from build123d import *

# Parameters (mm, degrees)
BOSS_EXTRU_1_DEPTH                      = 7
ESQUISSE2_R                             = 4
ESQUISSE2_R_2                           = 1.2
BOSS_EXTRU_2_DEPTH                      = 7
CONG_1_R                                = 10
CONG_2_R                                = 3
DIAM_TRE_DU_PER_AGE_2_4_2_4_1_D         = 2.4
DIAM_TRE_DU_PER_AGE_2_4_2_4_1_ON_FACE_D = 2.4
DIAM_TRE_DU_PER_AGE_2_4_2_4_1_ON_F_2_D  = 2.4


with BuildPart() as part:
    # Esquisse1 → Boss.-Extru.1 (new body)
    with BuildSketch(Plane(origin=(0, 0, 0), x_dir=(1, 0, 0), z_dir=(0, 1, 0))):
        with BuildLine():
            Line((163.5, -54.314885969), (163.5, 54.839745962))
            Line((163.5, 54.839745962), (123.5, 124.121778265))
            Line((123.5, 124.121778265), (119.169872981, 121.621778265))
            Line((119.169872981, 121.621778265), (158.5, 53.5))
            Line((158.5, 53.5), (158.5, -53.5))
            ThreePointArc((158.5, -53.5), (146.077391865, -81.52236249), (128.750264504, -106.807627959))
            Line((128.750264504, -106.807627959), (132.598479772, -110))
            ThreePointArc((132.598479772, -110), (150.644566487, -83.59767596), (163.5, -54.314885969))
        make_face()
    extrude(amount=BOSS_EXTRU_1_DEPTH)

    # Esquisse2 → Boss.-Extru.2 (add)
    # profile 1 of 2: a face of its own
    with BuildSketch(Plane(origin=(0, 7, 0), x_dir=(1, 0, 0), z_dir=(0, 1, 0))):
        with Locations((155, 53)):
            Circle(ESQUISSE2_R)
        with Locations(Location((155, 53, 0), (0, 0, 270))):
            Circle(ESQUISSE2_R_2, mode=Mode.SUBTRACT)
    # profile 2 of 2: a face of its own
    with BuildSketch(Plane(origin=(0, 7, 0), x_dir=(1, 0, 0), z_dir=(0, 1, 0))):
        with Locations((140, -87)):
            Circle(ESQUISSE2_R)
        with Locations(Location((140, -87, 0), (0, 0, 270))):
            Circle(ESQUISSE2_R_2, mode=Mode.SUBTRACT)
    extrude(amount=-BOSS_EXTRU_2_DEPTH)

    # Congé1
    cong_1_edges = [part.edges().sort_by_distance(p)[0] for p in [
        (158.5, 3.5, 53.5),
        (163.5, 3.5, -54.839745962),
        (163.5, 3.5, 54.314885969),
    ]]
    fillet(cong_1_edges, radius=CONG_1_R)

    # Congé2
    cong_2_edges = [part.edges().sort_by_distance(p)[0] for p in [
        (128.750264504, 3.5, 106.807627959),
        (119.169872981, 3.5, -121.621778265),
        (156.697559724, 3.5, -56.621918136),
        (158.5, 3.5, -51.063508327),
        (140.380940937, 3.5, 90.981819183),
        (143.738827918, 3.5, 85.578322891),
    ]]
    fillet(cong_2_edges, radius=CONG_2_R)

    # Diamètre du perçage Ø2.4 (2.4)1 (through all)
    with Locations(Plane(origin=(135.734675085, 4, 106.105866084), x_dir=(-0.615871636874, 0, 0.787846512269), z_dir=(0.787846512269, 0, 0.615871636874))):
        with Locations((0, 0)):
            Hole(DIAM_TRE_DU_PER_AGE_2_4_2_4_1_D / 2)

    # Diamètre du perçage Ø2.4 (2.4)1 on face (through all)
    with Locations(Plane(origin=(163.5, 4, -45), x_dir=(0, 0, 1), z_dir=(1, 0, 0))):
        with Locations((0, 0), (90, 0)):
            Hole(DIAM_TRE_DU_PER_AGE_2_4_2_4_1_ON_FACE_D / 2)

    # Diamètre du perçage Ø2.4 (2.4)1 on f 2 (through all)
    with Locations(Plane(origin=(126, 4, -119.791651246), x_dir=(0.500000174844, 0, 0.866025302838), z_dir=(0.866025302838, 0, -0.500000174844))):
        with Locations((0, 0)):
            Hole(DIAM_TRE_DU_PER_AGE_2_4_2_4_1_ON_F_2_D / 2)


solid = part.part
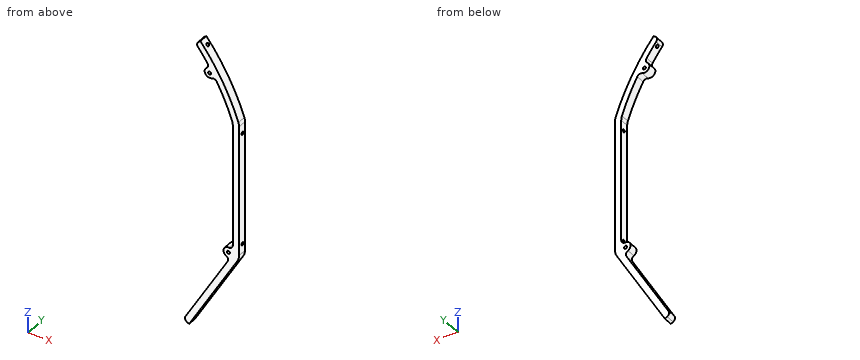
Part model, mm, in its own coordinate system. Coordinates: 2 decimals unless noted, no trailing zeros. Write each loop counter-clockwise with the first axis right and the second up, starting at its lowest first coordinate (ties: lowest second). Pieces come first, ordered by that corner, then holes. Notation, with made-up numbers: (-23.5, 46.25) - (20.5, 46.25) arc R18 ccw to (20.5, 63.25) - close; hole circle Ø8 at (89, -5). An arc over 180 degrees is marked (long way). Put each result on its own line as item: value.
1. Probe line 1 along X through (y, z) = (4.25, -53); line 2 along Z through (x, y) = (140, 1.25); line 3 along X through (y, z) = (5.75, 46.5). List the from-to ranges inside material, lowest first. Write a range as [from, to].
Final values:
line 1: x = [151, 153.8], [156.2, 163.46]
line 2: z = [-95.54, -85.54], [83, 85.8], [88.2, 100.41]
line 3: x = [158.5, 163.5]
2. Flat gauge pins, fed straight in: pin 1 Ø1.5 at (y, z) = (4, -72) entering from -X; pin 2 Ø2 at (x, y) = (130.5, 1.5) entering from +Z; pin 3 Ø2 at (x, y) = (157, 3.5) entering from -Z. Where does each tip first touch, or does it go through?
Final values:
pin 1: stops at x = 147.39
pin 2: stops at z = 109.09
pin 3: stops at z = -67.83
3. Band-saw the part on A-A (z = -18). Write the cut outline in (x, y), then the cut area to 3 significant figures.
Final values:
outline: (158.5, 0) - (163.5, 0) - (163.5, 7) - (158.5, 7) - close
area: 35.0 mm²
